Could you check a few things on this model? Use its own coordinates, in mm. Face numbers are marked on the shaded views. A direction names the side the tool comes from. Coordinates: 2 decimals unless noted, no trailing zeros. Order: outer loops, then holes, each group sorted by start corner. A loop starts at its lowest first (then second) coordinate and runs counter-clockwise, first axis right, second up. Notation, with made-up numbers: (62, 25) -> (74, 25) arc R24 ccw to (74, 55) -> close; hole circle Ø9 at (49, -34). An arc over 180 degrees is marked (long way). Use a Markdown table: item, result. Add a question column.
1) If we section it at A-A (z = 0): Write out the boundary of the cut face in (x, y).
2) If we section it at C-C (z = 15): Write out the boundary of the cut face in (x, y), plus the area to 3 significant figures.
3) If we section it at B-B (x = 81.5): Write out the boundary of the cut face in (y, z).
4) If I drill on L1, parallel to X at y = 14, z = 10.5; L2, parallel to Y at x = 20.75, z = 23.25; L3, parallel to Z at x = 1.8, y = 0, over which ranges is the centre line in solid material (lowest first)? Write a range as [from, to].
5) Which directions (+Z, -Z, +X, -X, +Y, -Y) give clear straight access to the entire face, cutting with the end or side of a thin tool? Please do the marked faces 1 and 2.
6) Will these pins go through, and if not, where does the flat tip stop? pin 1 Ø4 at (x, y) = (20.5, -16) entering from +Z; pin 2 Ø3.5 at (y, z) = (0, -10) entering from +X; pin 3 Ø4.5 at (x, z) = (107, 22) entering from -Y.
Autodesk Inventor part; units mm, degrees
ref_plane "YZ Plane" through (0, 0, 0) normal (1, 0, 0) x (0, 1, 0)
ref_plane "XZ Plane" through (0, 0, 0) normal (0, 1, 0) x (-1, 0, 0)
ref_plane "XY Plane" through (0, 0, 0) normal (0, 0, 1) x (1, 0, 0)
sketch "スケッチ1" plane through (0, 0, 0) normal (1, 0, 0) x (0, 1, 0)
  circle A0 centre (0, 0) radius 10
  circle A1 centre (0, -10) radius 1.35
  circle A2 centre (8.6603, 5) radius 1.35
  circle A3 centre (-8.6603, 5) radius 1.35
  circle A4 centre (0, 0) radius 5
  line L0 (0, 0) -> (0, 50)
  circle A5 centre (0, 50) radius 22.5
  circle A6 centre (0, 0) radius 14
  line L1 (-14, 0) -> (-22.5, 50)
  line L2 (14, 0) -> (22.5, 50)
  line L3 (0, -14) -> (-11.62, -14)
  line L4 (-11.62, -14) -> (-14, 0)
  line L5 (0, -14) -> (11.62, -14)
  line L6 (11.62, -14) -> (14, 0)
  line L7 (0, 20) -> (-17.4, 20)
  line L8 (0, 20) -> (17.4, 20)
  dimension "d0" = 20
  dimension "d1" = 2.7
  dimension "d4" = 360
  dimension "d6" = 10
  dimension "d7" = 50
  dimension "d8" = 45
  dimension "d9" = 28
extrude "押し出し1" add sketch "スケッチ1" along normal blind 4 contours A0 A1 A3 A2 | A6 L6 L4 | A6 L1 L7 L0 | L0 L8 L2 A6 | L6 L5 A6 | A6 L3 L4
sketch "スケッチ2" plane through (0, -17.4, 20) normal (0, 0, 1) x (1, 0, 0)
  line L0 (0, 17.4) -> (30, 17.4)
  circle A0 centre (30, 17.4) radius 22.5
  circle A1 centre (30, 17.4) radius 18.5
  circle A2 centre (30, 17.4) radius 14
  circle A3 centre (48.5, 17.4) radius 1.35
  circle A4 centre (20.75, 33.4215) radius 1.35
  circle A5 centre (20.75, 1.3785) radius 1.35
  line L1 (0, 29.02) -> (0, 34.8)
  line L2 (0, 0) -> (0, 5.78)
  line L3 (0, 34.8) -> (0, 0)
  line L4 (4, 29.02) -> (4, 34.8)
  line L5 (4, 34.8) -> (7, 34.8)
  line L6 (7, 34.8) -> (30, 39.9)
  line L7 (4, 0) -> (4, 5.78)
  line L8 (4, 0) -> (7, 0)
  line L9 (7, 0) -> (30, -5.1)
  line L10 (4, 0) -> (0, 0)
  line L11 (0, 34.8) -> (4, 34.8)
  line L12 (0, 0) -> (0, 34.8)
  line L13 (0, 34.8) -> (4, 34.8)
  dimension "d14" = 37
  dimension "d12" = 30
  dimension "d13" = 45
  dimension "d15" = 28
  dimension "d16" = 2.7
  dimension "d19" = 360
  dimension "d21" = 3
  dimension "d22" = 3
extrude "押し出し2" add sketch "スケッチ2" along normal blind 4 contours L3 L1 L11 L5 L6 A0 L0 | L0 A0 L9 L8 L10 L2 L3 | A1 A4 A3 A5 | A0 L6 L9
fillet "フィレット1" radius 3 2 edges at (4, 0, 20) (0, 0, 24)
fillet "フィレット2" radius 3 2 edges at (2, -11.62, -14) (2, 11.62, -14)
sketch "スケッチ7" plane through (0, -17.4, 24) normal (0, 0, 1) x (1, 0, 0)
  circle A0 centre (30, 17.4) radius 14
  line L0 (30, 17.4) -> (187, 17.4)
  line L1 (30, 17.4) -> (187, 17.4) construction
  circle A1 centre (187, 17.4) radius 3.5
  circle A2 centre (187, 17.4) radius 10
  line L2 (187, 27.4) -> (50.1556, 27.4)
  arc A3 (30, -5.1) -> (30, 39.9) centre (30, 17.4) ccw
  line L3 (187, 27.4) -> (323.8444, 27.4) construction
  line L4 (187, 7.4) -> (50.1556, 7.4)
  point P0 (0, 17.4)
  dimension "d55" = 157
  dimension "d56" = 0
  dimension "d57" = 7
  dimension "d58" = 20
  dimension "d59" = 180
extrude "押し出し7" add sketch "スケッチ7" against normal blind 4 contours A3 L2 A2 L0 | L0 A2 L4 A3 | A2
fillet "フィレット3" radius 2 2 edges at (50.1556, 10, 22) (50.1556, -10, 22)
sketch "スケッチ8" plane through (0, -17.4, 24) normal (0, 0, 1) x (1, 0, 0)
  circle A0 centre (20.75, 33.4215) radius 1.35
  circle A1 centre (20.75, 33.4215) radius 2.5
  circle A2 centre (48.5, 17.4) radius 1.35
  circle A3 centre (48.5, 17.4) radius 2.5
  circle A4 centre (20.75, 1.3785) radius 1.35
  circle A5 centre (20.75, 1.3785) radius 2.5
  point P0 (0, 17.4)
  dimension "d63" = 5
  dimension "d64" = 5
  dimension "d65" = 5
extrude "押し出し8" cut sketch "スケッチ8" against normal blind 2 contours A0 | A1 | A3 | A4 | A5
properties part number "motor_holder_2" material "アルミニウム 6061"
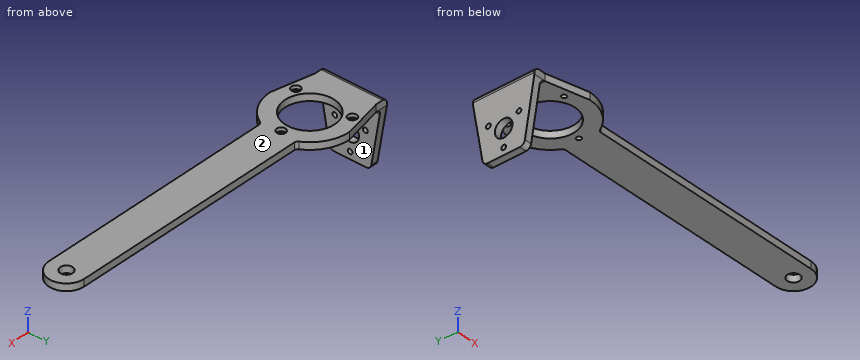
Answer sheet:
| question | item | result |
|---|---|---|
| 1 | outline | (0, -14) -> (4, -14) -> (4, -5) -> (0, -5) -> close; (0, 5) -> (4, 5) -> (4, 14) -> (0, 14) -> close |
| 2 | outline | (0, -16.55) -> (4, -16.55) -> (4, 16.55) -> (0, 16.55) -> close |
| 2 | area | 132 mm2 |
| 3 | outline | (-10, 20) -> (10, 20) -> (10, 24) -> (-10, 24) -> close |
| 4 | L1 | [0, 4] |
| 4 | L2 | [-20.45, -18.52], [-13.52, -10.51], [10.51, 13.52], [18.52, 20.45] |
| 4 | L3 | [-14, -11.35], [-8.65, -5], [5, 23.75] |
| 5 | face 1 | -Z, +X, +Y, -Y |
| 5 | face 2 | +Z, +X, -X, +Y, -Y |
| 6 | pin 1 | z = 22 |
| 6 | pin 2 | x = 4 |
| 6 | pin 3 | y = -10 |
